Could you check a few things on this model? Use its own coordinates, in mm. Coordinates: 2 decimals unless noted, no trailing zeros. Order: outer loops, then holes, each group sorted by start corner. A loop starts at its lowest first (then second) coordinate and runs counter-clockwise, first axis right, second up. Notation, with made-up numbers: (-40, 60) - (-2, 60) arc R22 ccw to (-2, 85) - close; hole circle Ø9 at (-16.5, 23). An arc over 180 degrees is marked (long way). Answer as a JSON object with one key per item and string values. Group by question number.
(1) Imagine slicing it at A-A, the plane x = 226.5. Write out the boundary of the cut face in (y, z).
(2) Imagine slicing it at B-B, the plane y = 55.5. Write out the boundary of the cut face in (x, z).
(3) Please list where these lines run through material, in increasing order: probe 1 along Y at (x, z) = (277, 1.1); probe 2 along Y at (x, z) = (195, 1.35); probe 3 along X at (y, z) = (23, 0.1).
(4) We'd pull the mould along X, two halves only. Please class faces 1 (the cylindrical face through (217.31, 73.76, 0.79)), 2 (the flat face through (235, 65, 0)): pulls with the +X half, pulls with the -X half, needs draft (parallel to the pull), parting line crosses it, or undercut.
(5) Will this pin go through, and if not, where does the flat tip stop? P1, Ø5, axis at x = 239, y = 105, coming from the -Z side.
(6) Imagine slicing it at C-C, the plane z = 1.05. Give the number of separate pieces and of enclosed holes in the cut face, and give its area (3 significant figures).
from build123d import *

# Parameters (mm, degrees)
F0_W     = 105.460206
F0_H     = 106.09659
F1_DEPTH = 1.6


with BuildPart() as f1:
    # F0 (on Top) → F1 (new body)
    with BuildSketch(Plane.XY):
        with Locations((236.142386, 64.362091)):
            Rectangle(F0_W, F0_H)
        with BuildLine():
            Line((192.937283, 35.55936), (195.399541, 35.55936))
            ThreePointArc((195.399541, 35.55936), (199.093456, 27.759301), (206.893515, 24.065386))
            Line((206.893515, 24.065386), (206.893515, 20.838796))
            Line((206.893515, 20.838796), (192.937283, 20.838796))
            Line((192.937283, 20.838796), (192.937283, 35.55936))
        make_face(mode=Mode.SUBTRACT)
        with BuildLine():
            Line((234.833515, 20.838796), (209.433515, 20.838796))
            Line((209.433515, 20.838796), (209.433515, 24.065386))
            ThreePointArc((209.433515, 24.065386), (217.233573, 27.759301), (220.927489, 35.55936))
            Line((220.927489, 35.55936), (223.339541, 35.55936))
            ThreePointArc((223.339541, 35.55936), (227.033456, 27.759301), (234.833515, 24.065386))
            Line((234.833515, 24.065386), (234.833515, 20.838796))
        make_face(mode=Mode.SUBTRACT)
        with BuildLine():
            Line((206.893515, 52.005386), (206.893515, 49.593334))
            ThreePointArc((206.893515, 49.593334), (199.099195, 45.905154), (195.401158, 38.115505))
            Line((195.401158, 38.115505), (192.937283, 38.115505))
            Line((192.937283, 38.115505), (192.937283, 63.49936))
            Line((192.937283, 63.49936), (195.399541, 63.49936))
            ThreePointArc((195.399541, 63.49936), (199.093456, 55.699301), (206.893515, 52.005386))
        make_face(mode=Mode.SUBTRACT)
        with BuildLine():
            Line((223.341158, 38.115505), (220.925872, 38.115505))
            ThreePointArc((220.925872, 38.115505), (217.227835, 45.905154), (209.433515, 49.593334))
            Line((209.433515, 49.593334), (209.433515, 52.005386))
            ThreePointArc((209.433515, 52.005386), (217.233573, 55.699301), (220.927489, 63.49936))
            Line((220.927489, 63.49936), (223.339541, 63.49936))
            ThreePointArc((223.339541, 63.49936), (227.033456, 55.699301), (234.833515, 52.005386))
            Line((234.833515, 52.005386), (234.833515, 49.593334))
            ThreePointArc((234.833515, 49.593334), (227.039195, 45.905154), (223.341158, 38.115505))
        make_face(mode=Mode.SUBTRACT)
        with BuildLine():
            Line((237.373515, 20.838796), (237.373515, 24.065386))
            ThreePointArc((237.373515, 24.065386), (245.173573, 27.759301), (248.867489, 35.55936))
            Line((248.867489, 35.55936), (251.279541, 35.55936))
            ThreePointArc((251.279541, 35.55936), (254.973456, 27.759301), (262.773515, 24.065386))
            Line((262.773515, 24.065386), (262.773515, 20.838796))
            Line((262.773515, 20.838796), (237.373515, 20.838796))
        make_face(mode=Mode.SUBTRACT)
        with BuildLine():
            Line((265.313515, 20.838796), (265.313515, 24.065386))
            ThreePointArc((265.313515, 24.065386), (273.113573, 27.759301), (276.807489, 35.55936))
            Line((276.807489, 35.55936), (279.347489, 35.55936))
            Line((279.347489, 35.55936), (279.347489, 20.838796))
            Line((279.347489, 20.838796), (265.313515, 20.838796))
        make_face(mode=Mode.SUBTRACT)
        with BuildLine():
            Line((251.281158, 38.115505), (248.865872, 38.115505))
            ThreePointArc((248.865872, 38.115505), (245.167835, 45.905154), (237.373515, 49.593334))
            Line((237.373515, 49.593334), (237.373515, 52.005386))
            ThreePointArc((237.373515, 52.005386), (245.173573, 55.699301), (248.867489, 63.49936))
            Line((248.867489, 63.49936), (251.279541, 63.49936))
            ThreePointArc((251.279541, 63.49936), (254.973456, 55.699301), (262.773515, 52.005386))
            Line((262.773515, 52.005386), (262.773515, 49.593334))
            ThreePointArc((262.773515, 49.593334), (254.979195, 45.905154), (251.281158, 38.115505))
        make_face(mode=Mode.SUBTRACT)
        with BuildLine():
            Line((279.347489, 38.09936), (276.807489, 38.09936))
            ThreePointArc((276.807489, 38.09936), (273.113573, 45.899419), (265.313515, 49.593334))
            Line((265.313515, 49.593334), (265.313515, 52.005386))
            ThreePointArc((265.313515, 52.005386), (273.113573, 55.699301), (276.807489, 63.49936))
            Line((276.807489, 63.49936), (279.347489, 63.49936))
            Line((279.347489, 63.49936), (279.347489, 38.09936))
        make_face(mode=Mode.SUBTRACT)
        with BuildLine():
            Line((206.893515, 79.945386), (206.893515, 77.533334))
            ThreePointArc((206.893515, 77.533334), (199.099195, 73.845154), (195.401158, 66.055505))
            Line((195.401158, 66.055505), (192.937283, 66.055505))
            Line((192.937283, 66.055505), (192.937283, 91.43936))
            Line((192.937283, 91.43936), (195.399541, 91.43936))
            ThreePointArc((195.399541, 91.43936), (199.093456, 83.639301), (206.893515, 79.945386))
        make_face(mode=Mode.SUBTRACT)
        with BuildLine():
            Line((223.341158, 66.055505), (220.925872, 66.055505))
            ThreePointArc((220.925872, 66.055505), (217.227835, 73.845154), (209.433515, 77.533334))
            Line((209.433515, 77.533334), (209.433515, 79.945386))
            ThreePointArc((209.433515, 79.945386), (217.233573, 83.639301), (220.927489, 91.43936))
            Line((220.927489, 91.43936), (223.339541, 91.43936))
            ThreePointArc((223.339541, 91.43936), (227.033456, 83.639301), (234.833515, 79.945386))
            Line((234.833515, 79.945386), (234.833515, 77.533334))
            ThreePointArc((234.833515, 77.533334), (227.039195, 73.845154), (223.341158, 66.055505))
        make_face(mode=Mode.SUBTRACT)
        with BuildLine():
            Line((206.893515, 107.885386), (206.893515, 105.473334))
            ThreePointArc((206.893515, 105.473334), (199.099195, 101.785154), (195.401158, 93.995505))
            Line((195.401158, 93.995505), (192.937283, 93.995505))
            Line((192.937283, 93.995505), (192.937283, 107.885386))
            Line((192.937283, 107.885386), (206.893515, 107.885386))
        make_face(mode=Mode.SUBTRACT)
        with BuildLine():
            Line((223.341158, 93.995505), (220.925872, 93.995505))
            ThreePointArc((220.925872, 93.995505), (217.227835, 101.785154), (209.433515, 105.473334))
            Line((209.433515, 105.473334), (209.433515, 107.885386))
            Line((209.433515, 107.885386), (234.833515, 107.885386))
            Line((234.833515, 107.885386), (234.833515, 105.473334))
            ThreePointArc((234.833515, 105.473334), (227.039195, 101.785154), (223.341158, 93.995505))
        make_face(mode=Mode.SUBTRACT)
        with BuildLine():
            Line((251.281158, 66.055505), (248.865872, 66.055505))
            ThreePointArc((248.865872, 66.055505), (245.167835, 73.845154), (237.373515, 77.533334))
            Line((237.373515, 77.533334), (237.373515, 79.945386))
            ThreePointArc((237.373515, 79.945386), (245.173573, 83.639301), (248.867489, 91.43936))
            Line((248.867489, 91.43936), (251.279541, 91.43936))
            ThreePointArc((251.279541, 91.43936), (254.973456, 83.639301), (262.773515, 79.945386))
            Line((262.773515, 79.945386), (262.773515, 77.533334))
            ThreePointArc((262.773515, 77.533334), (254.979195, 73.845154), (251.281158, 66.055505))
        make_face(mode=Mode.SUBTRACT)
        with BuildLine():
            Line((279.347489, 66.03936), (276.807489, 66.03936))
            ThreePointArc((276.807489, 66.03936), (273.113573, 73.839419), (265.313515, 77.533334))
            Line((265.313515, 77.533334), (265.313515, 79.945386))
            ThreePointArc((265.313515, 79.945386), (273.113573, 83.639301), (276.807489, 91.43936))
            Line((276.807489, 91.43936), (279.347489, 91.43936))
            Line((279.347489, 91.43936), (279.347489, 66.03936))
        make_face(mode=Mode.SUBTRACT)
        with BuildLine():
            Line((251.281158, 93.995505), (248.865872, 93.995505))
            ThreePointArc((248.865872, 93.995505), (245.167835, 101.785154), (237.373515, 105.473334))
            Line((237.373515, 105.473334), (237.373515, 107.885386))
            Line((237.373515, 107.885386), (262.773515, 107.885386))
            Line((262.773515, 107.885386), (262.773515, 105.473334))
            ThreePointArc((262.773515, 105.473334), (254.979195, 101.785154), (251.281158, 93.995505))
        make_face(mode=Mode.SUBTRACT)
        with BuildLine():
            Line((279.347489, 93.97936), (276.807489, 93.97936))
            ThreePointArc((276.807489, 93.97936), (273.113573, 101.779419), (265.313515, 105.473334))
            Line((265.313515, 105.473334), (265.313515, 107.885386))
            Line((265.313515, 107.885386), (279.347489, 107.885386))
            Line((279.347489, 107.885386), (279.347489, 93.97936))
        make_face(mode=Mode.SUBTRACT)
    extrude(amount=F1_DEPTH)


solid = f1.part
Result set:
{
 "1": {"outline": "(11.31, 0) - (20.84, 0) - (20.84, 1.6) - (11.31, 1.6) - close; (28.33, 0) - (45.33, 0) - (45.33, 1.6) - (28.33, 1.6) - close; (56.27, 0) - (73.27, 0) - (73.27, 1.6) - (56.27, 1.6) - close; (84.21, 0) - (101.21, 0) - (101.21, 1.6) - (84.21, 1.6) - close; (107.89, 0) - (117.41, 0) - (117.41, 1.6) - (107.89, 1.6) - close"},
 "2": {"outline": "(183.41, 0) - (192.94, 0) - (192.94, 1.6) - (183.41, 1.6) - close; (199.3, 0) - (217.03, 0) - (217.03, 1.6) - (199.3, 1.6) - close; (227.24, 0) - (244.97, 0) - (244.97, 1.6) - (227.24, 1.6) - close; (255.18, 0) - (272.91, 0) - (272.91, 1.6) - (255.18, 1.6) - close; (279.35, 0) - (288.87, 0) - (288.87, 1.6) - (279.35, 1.6) - close"},
 "3": {"probe 1": "y = 11.31 to 20.84, 35.56 to 38.1, 63.5 to 66.04, 91.44 to 93.98, 107.89 to 117.41", "probe 2": "y = 11.31 to 20.84, 35.56 to 38.12, 63.5 to 66.06, 91.44 to 94, 107.89 to 117.41", "probe 3": "x = 183.41 to 192.94, 206.89 to 209.43, 234.83 to 237.37, 262.77 to 265.31, 279.35 to 288.87"},
 "4": {"face 1": "undercut", "face 2": "needs draft"},
 "5": {"P1": "stops at z = 0"},
 "6": {"separate pieces": "1", "enclosed holes": "16", "area": "8,470 mm^2"}
}
